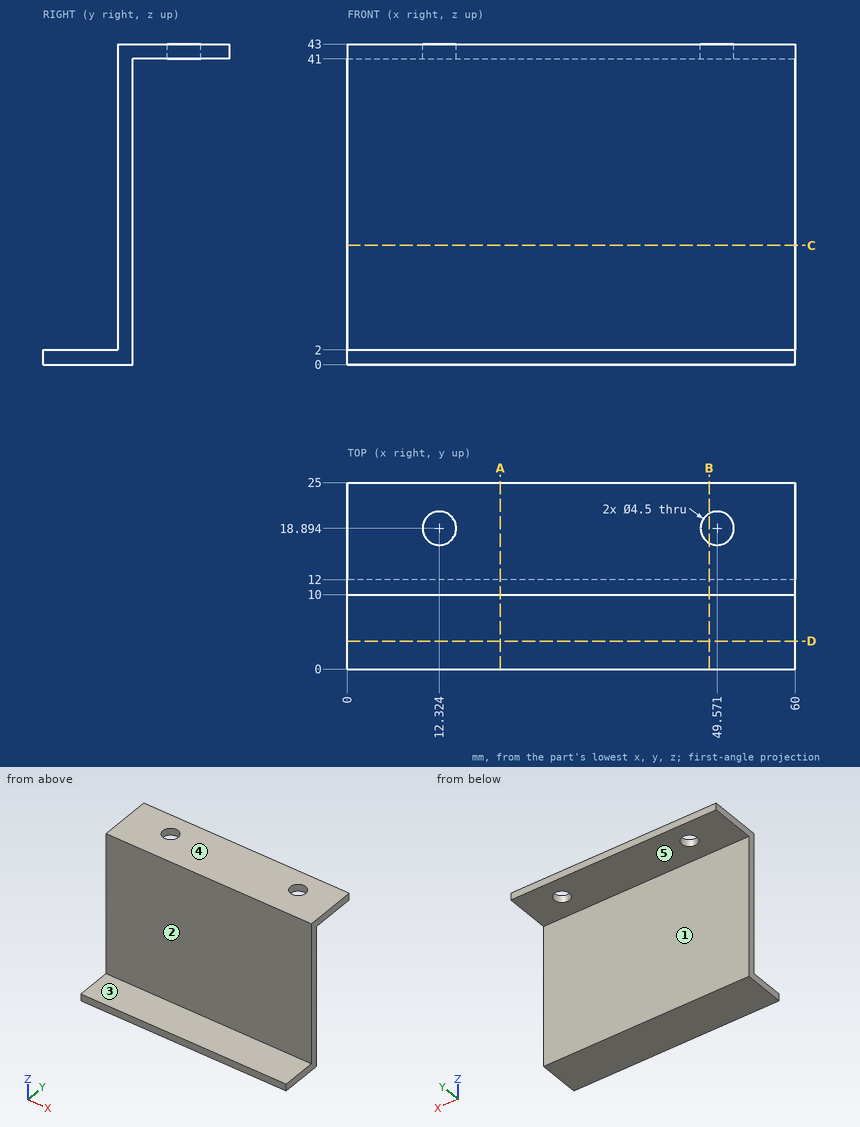
Geometry: see drawing. Coordinates: mm, zero at the bounding-box minimum. A direction names the side the tool comes from. Round coordinates to 2 decimals unless told otherwise and drop trailing zeros. Order: outer loops, then holes, each group sorted by start corner. A loop starts at its lowest first (then second) coordinate and runs counter-clockwise, first axis right, second up. Notation, with made-up numbers: (11.5, -39.5) - (18.5, -39.5) arc R30 cw to (18.5, -11.5) - close; hole circle Ø2 at (30, 35). An arc over 180 degrees is marked (long way). Use a Markdown table: item, result. Add a question column.
1. Set-up query: the marked faces 4 and 5. Return all of +Z, -Z, +X, -X, +Y, -Y with unobstructed straight access to the full face (end or side cutting, diameter ignored); none if empty.
2. Section query C-C (z = 16). Return the cut outline in (x, y).
3. Line query: probe 1 along Y at (x, z) = (4.5, 14); probe 2 along Z at (x, y) = (22.5, 14.75); probe 3 along Z at (x, y) = (41, 6.25). Output: solid intervals per line, ascending.
4. Section query A-A (x = 20.5). Return the cut outline in (y, z).
5. Mould query, pull axis Y, two halves, no side actions, for the marked faces 1, 2 and 3. Classes: +Y half, -Y half, draft (parallel to the pull), parting line (faces both ways), or undercut.
6. First-contact query: pin 1 (10 mm diameter, centred on y = 4, z = 35.5, fed in from -X); pin 2 (5 mm diameter, centred on x = 49.57, y = 18.89, fed in from -Z); pin 3 (5 mm diameter, centred on x = 50, y = 4.5, fed in from +Z); pin 4 (12.5 mm diameter, centred on x = 32, z = 11, fed in from +Y). Flat tips, straight axial feed; report the tip coordinate or a pass-through.
7. Section query D-D (y = 3.75). Return the cut outline in (x, z), then the cut area to 3 significant figures.
8. Section query B-B (x = 48.5). Return the cut outline in (y, z) (1 decimal).
Derived:
| question | item | result |
|---|---|---|
| 1 | face 4 | +Z, +X, -X, +Y, -Y |
| 1 | face 5 | -Z, +X, -X, +Y |
| 2 | outline | (0, 10) - (60, 10) - (60, 12) - (0, 12) - close |
| 3 | probe 1 | 10 to 12 |
| 3 | probe 2 | 41 to 43 |
| 3 | probe 3 | 0 to 2 |
| 4 | outline | (0, 0) - (12, 0) - (12, 41) - (25, 41) - (25, 43) - (10, 43) - (10, 2) - (0, 2) - close |
| 5 | face 1 | +Y half |
| 5 | face 2 | -Y half |
| 5 | face 3 | draft |
| 6 | pin 1 | through |
| 6 | pin 2 | z = 41 |
| 6 | pin 3 | z = 2 |
| 6 | pin 4 | y = 12 |
| 7 | outline | (0, 0) - (60, 0) - (60, 2) - (0, 2) - close |
| 7 | area | 120 mm2 |
| 8 | outline | (0, 0) - (12, 0) - (12, 41) - (16.9, 41) - (16.9, 43) - (10, 43) - (10, 2) - (0, 2) - close; (20.9, 41) - (25, 41) - (25, 43) - (20.9, 43) - close |
